Model file for the job. Use its own axes, mm. A direction names the side the tool comes from. Give positions to 0.01 mm unless a question says otherwise; leave off trailing zeros. Write each loop counter-clockwise with the first axis right and the second up, starting at its lowest first coordinate (ties: lowest second). Pieces come first, ordered by that corner, then holes.
```python
from build123d import *

# Parameters (mm, degrees)
SKETCH1_W           = 60
SKETCH1_H           = 90
BOSS_EXTRUDE1_DEPTH = 10
SKETCH2_R           = 30
BOSS_EXTRUDE2_DEPTH = 30
SKETCH6_R           = 8
BOSS_EXTRUDE3_DEPTH = 15


with BuildPart() as part:
    # Sketch1 → Boss-Extrude1 (new body)
    with BuildSketch(Plane.XY):
        Rectangle(SKETCH1_W, SKETCH1_H)
    extrude(amount=BOSS_EXTRUDE1_DEPTH)

    # Sketch2 → Boss-Extrude2 (add)
    with BuildSketch(Plane(origin=(0, 0, 0), x_dir=(-1, 0, 0), z_dir=(0, 0, -1))):
        Circle(SKETCH2_R)
        with BuildLine():
            Line((4, -13.912685387), (4, -13.325269778))
            ThreePointArc((4, -13.325269778), (0, 13.912685387), (-4, -13.325269778))
            Line((-4, -13.325269778), (-4, -13.912685387))
            Line((-4, -13.912685387), (-4, -16.912685387))
            Line((-4, -16.912685387), (4, -16.912685387))
            Line((4, -16.912685387), (4, -13.912685387))
        make_face(mode=Mode.SUBTRACT)
    extrude(amount=BOSS_EXTRUDE2_DEPTH)

    # Sketch6 → Boss-Extrude3 (add)
    with BuildSketch(Plane(origin=(0, 45, 0), x_dir=(1, 0, 0), z_dir=(0, 1, 0))):
        with BuildLine():
            Line((-30, -10), (-22.306028796, -40.607234555))
            ThreePointArc((-22.306028796, -40.607234555), (0, -58), (22.306028796, -40.607234555))
            Line((22.306028796, -40.607234555), (30, -10))
            Line((30, -10), (-30, -10))
        make_face()
        with Locations(Location((0, -35, 0), (0, 0, 270))):
            Circle(SKETCH6_R, mode=Mode.SUBTRACT)
    boss_extrude3 = extrude(amount=-BOSS_EXTRUDE3_DEPTH)

    # Mirror1: Boss-Extrude3 across plane
    add(boss_extrude3.mirror(Plane.ZX))


solid = part.part
```
1. Slice it at B-B, the plane z = 35. Write the cut outline in (x, y), and give its area (3 significant figures).
Calculated:
outline: (-23.72, -45) - (-8, -45) - (-8, -30) - (-23.72, -30) - close; (-23.72, 30) - (-8, 30) - (-8, 45) - (-23.72, 45) - close; (8, -45) - (23.72, -45) - (23.72, -30) - (8, -30) - close; (8, 30) - (23.72, 30) - (23.72, 45) - (8, 45) - close
area: 943 mm2
2. Pin check, flat tips, straight feed: P1, Ø3, axis at y = -14.5, z = -21, coming from the +X side; P2, Ø4, axis at x = 1, z = -18.5, coming from the +Y side; P3, Ø1, axis at x = -10, y = 18, coming from the +Z side. Stop position of each tip, or through.
Calculated:
P1: stops at x = 27.04
P2: stops at y = 30
P3: stops at z = 10
3. Slice it at A-A, the plane x = 0. Write the cut outline in (y, z), and give its area (3 significant figures).
Calculated:
outline: (-45, 0) - (-30, 0) - (-30, -30) - (-16.91, -30) - (-16.91, 0) - (13.91, 0) - (13.91, -30) - (30, -30) - (30, 0) - (45, 0) - (45, 27) - (30, 27) - (30, 10) - (-30, 10) - (-30, 27) - (-45, 27) - close; (-45, 43) - (-30, 43) - (-30, 58) - (-45, 58) - close; (30, 43) - (45, 43) - (45, 58) - (30, 58) - close
area: 2,740 mm2
4. Pull direction X, two halves, no side cores. Call faces 4 (the flat face through (0, -45, 22)), 5 (the cylindrical face through (-4.868, 37.605, 28.651)), 6 (the flat face through (26.1, 37.61, 25.52)): +X half, -X half, draft (parallel to the pull), parting line (faces both ways), or undercut.
Calculated:
face 4: draft
face 5: undercut
face 6: +X half
5. Which spindle directions (+Z, -Z, +X, -X, +Y, -Y) get a long thin tool onto all of the face, cutting with end or side? Do faces 1 (the flat face through (6, -30, 28)), 2 (the cylindrical face through (-0.6, 13.9, -14.8)), 3 (the flat face through (0, -32, 0)). Say none if no direction does.
Calculated:
face 1: +Z, +X, -X
face 2: -Z
face 3: -Z, -Y
6. Slice it at C-C, the plane y = 33.5. Write the cut outline in (x, z), and give its area (3 significant figures).
Calculated:
outline: (-30, 0) - (30, 0) - (30, 10) - (22.31, 40.61) arc R23 ccw to (-22.31, 40.61) - (-30, 10) - close; hole circle Ø16 at (0, 35)
area: 2,580 mm2
7. Slice it at D-D, the plane y = 22. Write the cut outline in (x, z), and give its area (3 significant figures).
Calculated:
outline: (-30, 0) - (-20.4, 0) - (-20.4, -30) - (20.4, -30) - (20.4, 0) - (30, 0) - (30, 10) - (-30, 10) - close
area: 1,820 mm2
8. Probe probe 1 along Y at (x, z) = (-5.5, 54); probe 2 along Z at (x, y) = (6.5, -18.5); probe 3 along Z at (x, y) = (1.5, 39). List the from-to ranges inside material, lowest first.
Calculated:
probe 1: y = -45 to -30, 30 to 45
probe 2: z = -30 to 10
probe 3: z = 0 to 27.14, 42.86 to 57.95
